Could you check a few things on this model? Use its own coordinates, in mm. A direction names the side the tool comes from. Round coordinates to 2 decimals unless told otherwise and drop trailing zeros. Loops run counter-clockwise (first coordinate to the right, second up) from the corner with the lowest first, then second, coordinate; pieces in that order, holes last. Notation, with made-up numbers: (3, -14.75) -> (50, -14.75) arc R29 cw to (50, 16.25) -> close; hole circle Ø2 at (-38.5, 59.5). An arc over 180 degrees is marked (long way). One line per item, written item: value.
from build123d import *

# Parameters (mm, degrees)
BOSS_EXTRUDE1_DEPTH = 15
SKETCH2_W           = 15
SKETCH2_H           = 8.7
BOSS_EXTRUDE2_DEPTH = 12.5
SKETCH3_W           = 10
SKETCH3_H           = 15
BOSS_EXTRUDE3_DEPTH = 15.5
SKETCH5_W           = 15
SKETCH5_H           = 10
BOSS_EXTRUDE4_DEPTH = 20


with BuildPart() as part:
    # Sketch1 → Boss-Extrude1 (new body)
    with BuildSketch(Plane.XY):
        Polygon((-3.665803919, -0.605497889), (-3.665803919, 8.094502111), (-2.615803919, 7.044502111), (-1.965803919, 7.044502111), (-1.965803919, 9.144502111), (-0.354656646, 9.144502111), (2.234196081, 6.555649384), (2.234196081, 0.933354838), (-0.354656646, -1.655497889), (-1.965803919, -1.655497889), (-1.965803919, 0.444502111), (-2.615803919, 0.444502111), align=None)
    extrude(amount=BOSS_EXTRUDE1_DEPTH)

    # Sketch2 → Boss-Extrude2 (add)
    with BuildSketch(Plane.ZY.offset(3.665803919)):
        with Locations((7.5, 3.744502111)):
            Rectangle(SKETCH2_W, SKETCH2_H)
    extrude(amount=BOSS_EXTRUDE2_DEPTH)

    # Sketch3 → Boss-Extrude3 (add)
    with BuildSketch(Plane(origin=(0, 8.094502111, 0), x_dir=(1, 0, 0), z_dir=(0, 1, 0))):
        with Locations((-11.165803919, -7.5)):
            Rectangle(SKETCH3_W, SKETCH3_H)
    extrude(amount=BOSS_EXTRUDE3_DEPTH)

    # Sketch5 → Boss-Extrude4 (add)
    with BuildSketch(Plane.ZY.offset(16.165803919)):
        with Locations((7.5, 18.594502111)):
            Rectangle(SKETCH5_W, SKETCH5_H)
    extrude(amount=BOSS_EXTRUDE4_DEPTH)


solid = part.part
(1) If we section it at B-B, the plane y = 0: Please give me the cut outline in (x, z).
Recorded:
outline: (-16.17, 0) -> (-3.06, 0) -> (-3.06, 15) -> (-16.17, 15) -> close; (-1.97, 0) -> (1.3, 0) -> (1.3, 15) -> (-1.97, 15) -> close
(2) If we section it at A-A, the plane z = 5: Please give me the cut outline in (x, y), then the cut area to 3 significant figures.
Recorded:
outline: (-36.17, 13.59) -> (-16.17, 13.59) -> (-16.17, -0.61) -> (-3.67, -0.61) -> (-2.62, 0.44) -> (-1.97, 0.44) -> (-1.97, -1.66) -> (-0.35, -1.66) -> (2.23, 0.93) -> (2.23, 6.56) -> (-0.35, 9.14) -> (-1.97, 9.14) -> (-1.97, 7.04) -> (-2.62, 7.04) -> (-3.67, 8.09) -> (-6.17, 8.09) -> (-6.17, 23.59) -> (-36.17, 23.59) -> close
area: 515 mm²
(3) For faces 1 (the face through (-1, 9.145, 7)), 2 (the face through (1, -0.3, 7.4)), 3 (the face through (-16.166, 6, 8)), 4 (the face through (-3.13, -0.07, 7.4)), 5 (the face through (-3.15, 7.58, 7.4)), which set-ups out of +Z, -Z, +X, -X, +Y, -Y let a thin tool reach every point of the face, with its end or its side?
Recorded:
face 1: +Z, -Z, +X, +Y
face 2: +Z, -Z, +X, -Y
face 3: +Z, -Z, -X, -Y
face 4: +Z, -Z, -Y
face 5: +Z, -Z, +Y
(4) I'm going to push flat-ended pins straight in: pin 1 Ø4 at (y, z) = (8.5, 6) entering from -X; pin 2 Ø3 at (x, z) = (-20, 5.5) entering from -Y; pin 3 Ø2 at (x, z) = (-5, 4.5) entering from +Y; pin 4 Ø10 at (x, y) = (-22, 10) entering from +Z. Where does each tip first touch, or does it pass through?
Recorded:
pin 1: x = -16.17
pin 2: y = 13.59
pin 3: y = 8.09
pin 4: z = 15
(5) If I drill on L1, parallel to X at y = 3, z = 12; L2, parallel to Y at x = -18.5, z = 13.5; L3, parallel to X at y = 10, z = 8.5, over which ranges is the centre line in solid material (lowest first)?
Recorded:
L1: -16.17 to 2.23
L2: 13.59 to 23.59
L3: -16.17 to -6.17
(6) If we section it at D-D, the plane y = 4.5: Please give me the cut outline in (x, z).
Recorded:
outline: (-16.17, 0) -> (2.23, 0) -> (2.23, 15) -> (-16.17, 15) -> close
(7) If we section it at C-C, the plane x = -18.5: Please give me the cut outline in (y, z).
Recorded:
outline: (13.59, 0) -> (23.59, 0) -> (23.59, 15) -> (13.59, 15) -> close
